Check sheet for the modelled part. Datum: model origin and axes. Units: mm. A direction names the side the tool comes from. Round coordinates to 2 decimals unless told otherwise and drop trailing zeros. Write each loop counter-clockwise with the first axis right and the second up, starting at its lowest first coordinate (ties: lowest second). Pieces come first, ordered by that corner, then holes. Notation, with made-up numbers: (-0.75, 27.5) -> (15.25, 27.5) arc R19 cw to (15.25, 38.5) -> close; hole circle Ø5 at (-13.75, 75.25). An arc over 180 degrees is marked (long way). One line per item, written item: value.
from build123d import *

# Parameters (mm, degrees)
SKETCH2_R                = 50
BOSS_EXTRUDE1_DEPTH      = 50
SKETCH3_R                = 13
BOSS_EXTRUDE2_DEPTH      = 12
SKETCH7_R                = 12
CUT_EXTRUDE3_DEPTH       = 12
SKETCH11_R               = 8.5
BOSS_EXTRUDE3_DEPTH      = 12
SKETCH12_R               = 7.5
CUT_EXTRUDE7_DEPTH       = 12
SKETCH15_R               = 2
CUT_EXTRUDE8_DEPTH       = 12
CUT_EXTRUDE8_DEPTH_BACK  = 12
SKETCH16_W               = 12
SKETCH16_H               = 5.5
CUT_EXTRUDE9_DEPTH       = 12
CUT_EXTRUDE9_DEPTH_BACK  = 12
SKETCH19_R               = 2
CUT_EXTRUDE12_DEPTH      = 16
CUT_EXTRUDE12_DEPTH_BACK = 16
SKETCH20_W               = 10
SKETCH20_H               = 12
CUT_EXTRUDE13_DEPTH      = 16
CUT_EXTRUDE13_DEPTH_BACK = 16
FILLET1_R                = 10


with BuildPart() as part:
    # Sketch2 → Boss-Extrude1 (new body)
    with BuildSketch(Plane.XY):
        Circle(SKETCH2_R)
    extrude(amount=BOSS_EXTRUDE1_DEPTH)

    # Sketch3 → Boss-Extrude2 (add)
    with BuildSketch(Plane(origin=(0, 0, 0), x_dir=(-1, 0, 0), z_dir=(0, 0, -1))):
        Circle(SKETCH3_R)
    extrude(amount=BOSS_EXTRUDE2_DEPTH)

    # Sketch7 → Cut-Extrude3 (cut)
    with BuildSketch(Plane(origin=(0, 0, -12), x_dir=(-1, 0, 0), z_dir=(0, 0, -1))):
        Circle(SKETCH7_R)
    extrude(amount=-CUT_EXTRUDE3_DEPTH, mode=Mode.SUBTRACT)

    # Sketch11 → Boss-Extrude3 (add)
    with BuildSketch(Plane.XY.offset(50)):
        Circle(SKETCH11_R)
    extrude(amount=BOSS_EXTRUDE3_DEPTH)

    # Sketch12 → Cut-Extrude7 (cut)
    with BuildSketch(Plane.XY.offset(62)):
        Circle(SKETCH12_R)
    extrude(amount=-CUT_EXTRUDE7_DEPTH, mode=Mode.SUBTRACT)

    # Sketch15 → Cut-Extrude8 (cut, two sides)
    with BuildSketch(Plane(origin=(0, 0, 0), x_dir=(0, 0, -1), z_dir=(1, 0, 0))) as cut_extrude8_sk:
        with Locations((-59.444436812, 0)):
            Circle(SKETCH15_R)
    extrude(amount=CUT_EXTRUDE8_DEPTH, mode=Mode.SUBTRACT)
    extrude(cut_extrude8_sk.sketch, amount=-CUT_EXTRUDE8_DEPTH_BACK, mode=Mode.SUBTRACT)

    # Sketch16 → Cut-Extrude9 (cut, two sides)
    with BuildSketch(Plane(origin=(0, 0, 0), x_dir=(0, 0, -1), z_dir=(1, 0, 0))) as cut_extrude9_sk:
        with Locations((-56, 5.75)):
            Rectangle(SKETCH16_W, SKETCH16_H)
        with Locations((-56, -5.75)):
            Rectangle(SKETCH16_W, SKETCH16_H)
    extrude(amount=CUT_EXTRUDE9_DEPTH, mode=Mode.SUBTRACT)
    extrude(cut_extrude9_sk.sketch, amount=-CUT_EXTRUDE9_DEPTH_BACK, mode=Mode.SUBTRACT)

    # Sketch19 → Cut-Extrude12 (cut, two sides)
    with BuildSketch(Plane(origin=(0, 0, 0), x_dir=(1, 0, 0), z_dir=(0, 1, 0))) as cut_extrude12_sk:
        with Locations((0, 7.94)):
            Circle(SKETCH19_R)
    extrude(amount=CUT_EXTRUDE12_DEPTH, mode=Mode.SUBTRACT)
    extrude(cut_extrude12_sk.sketch, amount=-CUT_EXTRUDE12_DEPTH_BACK, mode=Mode.SUBTRACT)

    # Sketch20 → Cut-Extrude13 (cut, two sides)
    with BuildSketch(Plane(origin=(0, 0, 0), x_dir=(1, 0, 0), z_dir=(0, 1, 0))) as cut_extrude13_sk:
        with Locations((-8, 6)):
            Rectangle(SKETCH20_W, SKETCH20_H)
        with Locations((8, 6)):
            Rectangle(SKETCH20_W, SKETCH20_H)
    extrude(amount=CUT_EXTRUDE13_DEPTH, mode=Mode.SUBTRACT)
    extrude(cut_extrude13_sk.sketch, amount=-CUT_EXTRUDE13_DEPTH_BACK, mode=Mode.SUBTRACT)

    # Fillet1
    fillet1_edges = [part.edges().sort_by_distance(p)[0] for p in [
        (-50, 0, 0),
        (-50, 0, 50),
    ]]
    fillet(fillet1_edges, radius=FILLET1_R)


solid = part.part
Item 1: Depth check by flat-ended pin: pin 1 (10 mm diameter, centred on y = -20.5, z = 46, fed in from -X); pin 2 (4 mm diameter, centred on x = 32.5, y = 0.5, fed in from +Z); pin 3 (1.1 mm diameter, centred on y = -12, z = -9, fed in from +X). Enter the tip coordinate at first touch or a pass-through.
Result set:
pin 1: x = -46.72
pin 2: z = 50
pin 3: x = 3
Item 2: Sectioned sample at C-C (z = -7.94). Enter the section's corners in (x, y).
Result set:
outline: (-3, -12.65) arc R13 ccw to (-2, -12.85) -> (-2, -11.83) arc R12 cw to (-3, -11.62) -> close; (-3, 11.62) arc R12 cw to (-2, 11.83) -> (-2, 12.85) arc R13 ccw to (-3, 12.65) -> close; (2, -12.85) arc R13 ccw to (3, -12.65) -> (3, -11.62) arc R12 cw to (2, -11.83) -> close; (2, 11.83) arc R12 cw to (3, 11.62) -> (3, 12.65) arc R13 ccw to (2, 12.85) -> close
Item 3: Release check for a two-part mould opening along X. For faces 6 (the flat face through (-1, 1, 0)), 7 (the cylindrical face through (1.847, 12.408, -7.174)), 8 (the cylindrical face through (-8.5, 0, 54.6)) record: pulls with the +X half, pulls with the -X half, needs draft (parallel to the pull), parting line crosses it, or undercut.
Result set:
face 6: needs draft
face 7: undercut
face 8: pulls with the -X half
Item 4: Sectioned sample at A-A (x = 0). Enter the section's corners in (y, z).
Result set:
outline: (-50, 10) arc R10 ccw to (-40, 0) -> (-13, 0) -> (-13, -5.94) -> (-12, -5.94) -> (-12, 0) -> (12, 0) -> (12, -5.94) -> (13, -5.94) -> (13, 0) -> (40, 0) arc R10 ccw to (50, 10) -> (50, 40) arc R10 ccw to (40, 50) -> (-40, 50) arc R10 ccw to (-50, 40) -> close; (-13, -12) -> (-12, -12) -> (-12, -9.94) -> (-13, -9.94) -> close; (12, -12) -> (13, -12) -> (13, -9.94) -> (12, -9.94) -> close
Item 5: Sectioned sample at D-D (z = 30). Enter the section's corners in (x, y).
Result set:
outline: circle Ø100 at (0, 0)
Item 6: Sectioned sample at B-B (y = 0). Enter the section's corners in (x, z), then the cut area to 3 significant figures.
Result set:
outline: (-50, 10) arc R10 ccw to (-40, 0) -> (40, 0) arc R10 ccw to (50, 10) -> (50, 40) arc R10 ccw to (40, 50) -> (8.5, 50) -> (8.5, 57.44) -> (7.5, 57.44) -> (7.5, 50) -> (-7.5, 50) -> (-7.5, 57.44) -> (-8.5, 57.44) -> (-8.5, 50) -> (-40, 50) arc R10 ccw to (-50, 40) -> close; (-8.5, 61.44) -> (-7.5, 61.44) -> (-7.5, 62) -> (-8.5, 62) -> close; (7.5, 61.44) -> (8.5, 61.44) -> (8.5, 62) -> (7.5, 62) -> close
area: 4,930 mm^2
Item 7: Tool access check on faces 1 (the cylindrical face through (8.5, 0, 54.6)), 2 (the cylindrical face through (0, 13, -5)), 3 (the cylindrical face through (0, 12, -5)), 4 (the cylindrical face through (0, -13, -5)), 5 (the cylindrical face through (7.5, 0, 56.1)). Record the directions out of +Z, -Z, +X, -X, +Y, -Y that give a thin tool (end or side, any length) a straight path to the whole face; none if there is none.
Result set:
face 1: +Z, +X
face 2: -Z, +Y
face 3: -Z
face 4: -Z, -Y
face 5: +Z
Item 8: Material ranges on line 1 along Z through (x, y) = (0, 12.3); line 2 along Z through (x, y) = (-5.5, 26); line 3 along X through (y, z) = (-12, -7), recorded low to high.
Result set:
line 1: -12 to -9.94, -5.94 to 50
line 2: 0 to 50
line 3: -3 to -1.77, 1.77 to 3
